Geometry: final body of the model. Coordinates: model frame, mm. A direction names the side the tool comes from. Give positions to 0.01 mm unless a question says otherwise; leave off trailing zeros. Write each loop counter-clockwise with the first axis right and the second up, starting at its lowest first coordinate (ties: lowest second). Pieces come first, ordered by that corner, then holes. Notation, with made-up numbers: M 15,-4 L 39,-4 A20 cw 39,5 Z; hole C -10,-4 d5. An arc over 180 degrees is marked long. Answer as a JSON object with one key per item and string values.
from build123d import *

# Parameters (mm, degrees)
F0_R     = 5
F0_R_2   = 6
F1_DEPTH = 12.5
F3_DEPTH = 12.5


with BuildPart() as f1:
    # F0 (on Front) → F1 (new body, symmetric)
    with BuildSketch(Plane.XZ):
        with BuildLine():
            ThreePointArc((10, 7.5), (11.858541, 3.952847), (12.5, 0))
            ThreePointArc((12.5, 0), (11.858541, -3.952847), (10, -7.5))
            Line((10, -7.5), (118.385622, -7.5))
            ThreePointArc((118.385622, -7.5), (115, 0), (118.385622, 7.5))
            Line((118.385622, 7.5), (10, 7.5))
        make_face()
        with BuildLine():
            ThreePointArc((135, 0), (129.114378, 9.114378), (118.385622, 7.5))
            ThreePointArc((118.385622, 7.5), (115, 0), (118.385622, -7.5))
            ThreePointArc((118.385622, -7.5), (129.114378, -9.114378), (135, 0))
        make_face()
        with Locations((125, 0)):
            Circle(F0_R, mode=Mode.SUBTRACT)
        with BuildLine():
            ThreePointArc((10, -7.5), (11.858541, -3.952847), (12.5, 0))
            ThreePointArc((12.5, 0), (11.858541, 3.952847), (10, 7.5))
            ThreePointArc((10, 7.5), (-12.5, 0), (10, -7.5))
        make_face()
        Circle(F0_R_2, mode=Mode.SUBTRACT)
    extrude(amount=F1_DEPTH, both=True)

    # F2 (on Top) → F3 (intersect, symmetric)
    with BuildSketch(Plane.XY):
        Polygon((27.408045, 0), (-19.638073, 0), (-19.638073, -10), (28.180582, -10), (95.801556, 0.51067), (143.513262, 0.51067), (143.513262, 10.51067), (95.029019, 10.51067), align=None)
    extrude(amount=F3_DEPTH, both=True, mode=Mode.INTERSECT)


solid = f1.part
1) Contact query for flat-ended pins moving along their axis: P1, Ø1, axis at y = -4.5, z = 8.5, coming from the -X side; P2, Ø6, axis at x = 109.5, z = -4, coming from the -Y side; P3, Ø6, axis at x = 88.5, y = 5.5, coming from the -Z side; P4, Ø9, axis at x = 125, z = 0, coming from the +Y side. Output: stop coordinate, or through.
Geometry check:
{"P1": "stops at x = -9.6", "P2": "stops at y = 0.51", "P3": "stops at z = -7.5", "P4": "passes through"}
2) Pull-direction query (Z, two-part tool) for faces 5 (the cylindrical face through (129.77, 5.58, 1.5)), 6 (the cylindrical face through (-12.492, -5.07, 0.437)), 7 (the flat face through (115, 10.511, 0)); classes: pulls with the +Z half, pulls with the -Z half, needs draft (parallel to the pull), parting line crosses it, or undercut.
Geometry check:
{"face 5": "undercut", "face 6": "parting line crosses it", "face 7": "needs draft"}
3) Cut plane D-D on z = 3.75. Return loops of the section in (x, y).
Geometry check:
{"outline": "M -11.92,-10 L -4.68,-10 L -4.68,0 L -11.92,0 Z; M 4.68,-10 L 28.18,-10 L 95.8,0.51 L 121.69,0.51 L 121.69,10.51 L 95.03,10.51 L 27.41,0 L 4.68,0 Z; M 128.31,0.51 L 134.27,0.51 L 134.27,10.51 L 128.31,10.51 Z"}
4) Line query: line 1 (Z direction, x = 125, y = 5.75); line 2 (Z direction, x = 0, y = -4.25); line 3 (Z direction, x = 15, y = -1.75). Output: solid intervals per line, ascending. Write a range as from..to.
Geometry check:
{"line 1": "z = -10..-5, 5..10", "line 2": "z = -12.5..-6, 6..12.5", "line 3": "z = -7.5..7.5"}
5) Cut plane A-A on x = 0. Return loops of the section in (y, z), and give its area (3 significant figures).
Geometry check:
{"outline": "M -10,-12.5 L 0,-12.5 L 0,-6 L -10,-6 Z; M -10,6 L 0,6 L 0,12.5 L -10,12.5 Z", "area": "130 mm2"}
6) Cut plane B-B on z = -3.5. Return loops of the section in (x, y).
Geometry check:
{"outline": "M -12,-10 L -4.87,-10 L -4.87,0 L -12,0 Z; M 4.87,-10 L 28.18,-10 L 95.8,0.51 L 121.43,0.51 L 121.43,10.51 L 95.03,10.51 L 27.41,0 L 4.87,0 Z; M 128.57,0.51 L 134.37,0.51 L 134.37,10.51 L 128.57,10.51 Z"}
7) Set-up query: faces 1 (the flat face through (115, 0.511, 0)), 2 (the flat face through (8, 0, 0)), 3 (the flat face through (63, 0, -7.5)), 4 (the flat face through (65, 0, 7.5)). Return all of +Z, -Z, +X, -X, +Y, -Y with unobstructed straight access to the full face (end or side cutting, diameter ignored); none if empty.
Geometry check:
{"face 1": "+Z, -Z, +X, -Y", "face 2": "+Z, -Z, -X, +Y", "face 3": "-Z, +Y, -Y", "face 4": "+Z, +Y, -Y"}
8) Cut plane C-C on y = 1.75. Return loops of the section in (x, z).
Geometry check:
{"outline": "M 38.67,-7.5 L 118.39,-7.5 A10 ccw long 118.39,7.5 L 38.67,7.5 Z; hole C 125,0 d10"}
